For this review, take the finished solid that the model builds, in its own axes (mm). A direction names the side the tool comes from. Coordinates: 2 decimals unless noted, no trailing zeros. Loops run counter-clockwise (first coordinate to the right, second up) from the corner with the lowest first, then second, coordinate; pieces in that order, holes last. Notation, with made-up numbers: (10.5, -2.5) -> (56.5, -2.5) arc R35 cw to (56.5, 35.5) -> close; hole circle Ø6 at (30.5, -17.75). An arc over 180 degrees is marked (long way). One line per item, written item: value.
from build123d import *

# Parameters (mm, degrees)
SKETCH_1_R               = 87.5
EXTRUDE_1_DEPTH          = 55
EXTRUDE_2_DEPTH          = 55
PATTERN_CIRCULAR_1_COUNT = 20
CUT_EXTRUDE_1_DEPTH      = 191.525588833


with BuildPart() as part:
    # 草图1 → 拉伸1 (new, symmetric)
    with BuildSketch(Plane.XY):
        Circle(SKETCH_1_R)
    extrude(amount=EXTRUDE_1_DEPTH, both=True)

    # 草图2 → 拉伸2 (add, symmetric)
    with BuildSketch(Plane.XY):
        with BuildLine():
            ThreePointArc((10, 86.926693254), (0, 87.5), (-10, 86.926693254))
            ThreePointArc((-10, 86.926693254), (-8.101258535, 98.817083904), (-3.5, 109.944304082))
            ThreePointArc((-3.5, 109.944304082), (0, 110), (3.5, 109.944304082))
            ThreePointArc((3.5, 109.944304082), (8.101258535, 98.817083904), (10, 86.926693254))
        make_face()
    extrude_2 = extrude(amount=EXTRUDE_2_DEPTH, both=True)

    # 阵列(圆周)1: 拉伸2 ×20 about axis
    pattern_circular_1_axis = Axis((0, 0, 0), (0, 0, 1))
    for i in range(1, PATTERN_CIRCULAR_1_COUNT):
        add(extrude_2.rotate(pattern_circular_1_axis, i * 360 / PATTERN_CIRCULAR_1_COUNT))

    # 草图3 → 切除-拉伸1 (cut, through all)
    with BuildSketch(Plane.XY.offset(-55)):
        with BuildLine():
            Line((57.827329179, 16), (67, 16))
            Line((67, 16), (67, -16))
            Line((67, -16), (57.827329179, -16))
            ThreePointArc((57.827329179, -16), (-60, 0), (57.827329179, 16))
        make_face()
    extrude(amount=CUT_EXTRUDE_1_DEPTH, mode=Mode.SUBTRACT)


solid = part.part
1. Take a section at A-A, the plane y = 0. Give the boundary of the cut face in (x, z).
Return value:
outline: (-110, -55) -> (-60, -55) -> (-60, 55) -> (-110, 55) -> close; (67, -55) -> (110, -55) -> (110, 55) -> (67, 55) -> close
2. For faces 4 (the cylindrical face through (61.909, 61.835, 0.77)), 5 (the cylindrical face through (-51.66, 84.81, 0.77)), 6 (the cylindrical face through (98.98, -8.055, 0.77)), 7 (the cylindrical face through (-96.343, 22.738, 0.77)), list the 3-axis set-ups (+Z, -Z, +X, -X, +Y, -Y) from which the entire face can be reached by the end or side of a thin tool; tool diameter is ignored.
Return value:
face 4: +Z, -Z
face 5: +Z, -Z, +Y
face 6: +Z, -Z, +X
face 7: +Z, -Z, -X
3. To check wall thickness, follow probe 1 along Y at (x, z) = (0, -28); probe 2 along X at (y, z) = (0, 8.5); probe 3 along Y at (x, z) = (81, -10.5). State the ranges of each line that lie inside material, in increasing order. Write a range as from..to.
Return value:
probe 1: y = -110..-60, 60..110
probe 2: x = -110..-60, 67..110
probe 3: y = -66.4..-47.32, -36.75..36.75, 47.32..66.4
4. The part is to be moulded in two halves that separate along Y. For faces 1 (the cylindrical face through (88.96, 64.7, 0.77)), 2 (the cylindrical face through (-64.695, -75.342, 0.77)), 3 (the cylindrical face through (-51.397, -84.602, 0.77)), say which applies: pulls with the +Y half, pulls with the -Y half, needs draft (parallel to the pull), parting line crosses it, or undercut.
Return value:
face 1: pulls with the +Y half
face 2: undercut
face 3: pulls with the -Y half
5. Take a section at B-B, the plane x = 0. Give the boundary of the cut face in (y, z), and give its area (3 significant figures).
Return value:
outline: (-110, -55) -> (-60, -55) -> (-60, 55) -> (-110, 55) -> close; (60, -55) -> (110, -55) -> (110, 55) -> (60, 55) -> close
area: 11,000 mm2
6. Insertion check: pin 1 Ø5 at (x, z) = (3, -42) entering from +Y; pin 2 Ø4 at (x, z) = (-27, 1) entering from -Y; pin 3 Ø10 at (x, z) = (64.5, 23) entering from +Y; pin 4 Ø3 at (x, y) = (87, 41) entering from +Z. Each pin has a flat end and moves straight along its axis. Give the tip position at first contact, or say it passes through.
Return value:
pin 1: stops at y = 110
pin 2: stops at y = -104.05
pin 3: stops at y = 91
pin 4: passes through
